```python
from build123d import *

# Parameters (mm, degrees)
SKETCH1_R           = 3.175
SKETCH1_R_2         = 11
BOSS_EXTRUDE1_DEPTH = 10
FILLET3_R           = 2


with BuildPart() as part:
    # Sketch1 → Boss-Extrude1 (new body)
    with BuildSketch(Plane.XY):
        with BuildLine():
            Line((-69.85, -12.7), (-69.85, 12.7))
            Line((-69.85, 12.7), (61.868145579, 12.7))
            ThreePointArc((61.868145579, 12.7), (64.505886278, 14.015721477), (67.35, 14.790199458))
            Line((67.35, 14.790199458), (72.35, 14.790199458))
            ThreePointArc((72.35, 14.790199458), (84.85, 0), (72.35, -14.790199458))
            Line((72.35, -14.790199458), (67.35, -14.790199458))
            ThreePointArc((67.35, -14.790199458), (64.505886278, -14.015721477), (61.868145579, -12.7))
            Line((61.868145579, -12.7), (-69.85, -12.7))
        make_face()
        with Locations((-57.15, 0)):
            Circle(SKETCH1_R, mode=Mode.SUBTRACT)
        with Locations((69.85, 0)):
            Circle(SKETCH1_R_2, mode=Mode.SUBTRACT)
        with BuildLine():
            Line((-31.75, 3.175), (44.45, 3.175))
            ThreePointArc((44.45, 3.175), (47.625, 0), (44.45, -3.175))
            Line((44.45, -3.175), (-31.75, -3.175))
            ThreePointArc((-31.75, -3.175), (-34.925, 0), (-31.75, 3.175))
        make_face(mode=Mode.SUBTRACT)
    extrude(amount=BOSS_EXTRUDE1_DEPTH)

    # Fillet3
    fillet3_edges = [part.edges().sort_by_distance(p)[0] for p in [
        (-69.85, -12.7, 5),
        (-69.85, 12.7, 5),
    ]]
    fillet(fillet3_edges, radius=FILLET3_R)


solid = part.part
```
Can you work these out from the model? Positions are in its coordinate system, mm. A direction names the side the tool comes from. Give positions to 0.01 mm unless a question says otherwise; leave off trailing zeros. Loops run counter-clockwise (first coordinate to the right, second up) from the corner with the lowest first, then second, coordinate; pieces in that order, holes last. Notation, with made-up numbers: M 5,-21.75 L 62,-21.75 A14 ccw 62,-12.75 Z; hole C 87,59.25 d1. An arc over 180 degrees is marked long. Answer in a Markdown table with one row per item.
1. Suppose I cut it at A-A on y = 0. Write out the boundary of the cut face in (x, z) (3 decimals).
Taken from the geometry:
| item | result |
|---|---|
| outline | M -69.85,0 L -60.325,0 L -60.325,10 L -69.85,10 Z; M -53.975,0 L -34.925,0 L -34.925,10 L -53.975,10 Z; M 47.625,0 L 58.85,0 L 58.85,10 L 47.625,10 Z; M 80.85,0 L 84.85,0 L 84.85,10 L 80.85,10 Z |
2. Which directions (+Z, -Z, +X, -X, +Y, -Y) give clear straight access to the entire face, cutting with the end or side of a thin tool? Please do faces 1 (the flat face through (6, 3.175, 5)), 2 (the flat face through (-69.85, 0, 5)), 3 (the flat face through (-2, -12.7, 5)), 4 (the flat face through (-4, 12.7, 5)).
Taken from the geometry:
| item | result |
|---|---|
| face 1 | +Z, -Z |
| face 2 | +Z, -Z, -X, +Y, -Y |
| face 3 | +Z, -Z, -X, -Y |
| face 4 | +Z, -Z, -X, +Y |
3. Thinking about a two-plate mould opening in X: for faces 5 (the flat face through (70, -14.79, 5)), 6 (the cylindrical face through (-54.12, 0.95, 4.93)), 7 (the cylindrical face through (84.847, 0.295, 4.93)), 8 (the cylindrical face through (64.47, 14, 4.93)), which applies, released by +X, released by -X, zero draft, split by the parting line, or undercut?
Taken from the geometry:
| item | result |
|---|---|
| face 5 | zero draft |
| face 6 | undercut |
| face 7 | released by +X |
| face 8 | released by -X |
4. Suppose I cut it at C-C on z = 3.25. Write out the boundary of the cut face in (x, y) (3 decimals).
Taken from the geometry:
| item | result |
|---|---|
| outline | M -69.85,-10.7 A2 ccw -67.85,-12.7 L 61.868,-12.7 A15 ccw 67.35,-14.79 L 72.35,-14.79 A15 ccw 72.35,14.79 L 67.35,14.79 A15 ccw 61.868,12.7 L -67.85,12.7 A2 ccw -69.85,10.7 Z; hole C -57.15,0 d6.35; hole M -31.75,-3.175 L 44.45,-3.175 A3.175 ccw 44.45,3.175 L -31.75,3.175 A3.175 ccw Z; hole C 69.85,0 d22 |
5. For pin 1 Ø4 at (y, z) = (4.5, 1.5) entering from +X; pin 2 Ø4 at (x, z) = (13.5, 7.5) entering from -Y; pin 3 Ø3 at (x, z) = (8.5, 5) entering from +Y, each with a flat end and sliding along its axis, tell me the tip position at first contact or that it passes through.
Taken from the geometry:
| item | result |
|---|---|
| pin 1 | stops at x = 84.64 |
| pin 2 | stops at y = -12.7 |
| pin 3 | stops at y = 12.7 |
6. Suppose I cut it at B-B on x = 69.85. Write out the boundary of the cut face in (y, z).
Taken from the geometry:
| item | result |
|---|---|
| outline | M -14.79,0 L -11,0 L -11,10 L -14.79,10 Z; M 11,0 L 14.79,0 L 14.79,10 L 11,10 Z |
7. If I drill on line 1 along Y through (x, z) = (33, 8) (3 decimals); line 2 along Y through (x, z) = (69.85, 5.5); line 3 along X through (y, z) = (4.25, 4), over which ranges is the centre line in solid material (lowest first)?
Taken from the geometry:
| item | result |
|---|---|
| line 1 | y = -12.7 to -3.175, 3.175 to 12.7 |
| line 2 | y = -14.79 to -11, 11 to 14.79 |
| line 3 | x = -69.85 to 59.7, 80 to 84.24 |
8. Suppose I cut it at D-D on x = -18. Write out the boundary of the cut face in (y, z) (3 decimals).
Taken from the geometry:
| item | result |
|---|---|
| outline | M -12.7,0 L -3.175,0 L -3.175,10 L -12.7,10 Z; M 3.175,0 L 12.7,0 L 12.7,10 L 3.175,10 Z |
